Build history of the part. All positions in model axes, mm. Give positions to 0.01 mm unless a question says otherwise; leave off trailing zeros. Order: outer loops, then holes, each group sorted by start corner. A loop starts at its lowest first (then second) coordinate and runs counter-clockwise, first axis right, second up. Notation, with made-up numbers: (-23, 2) - (9, 2) arc R14 ccw to (9, 8) - close; hole circle Ø11 at (26.5, 38.5). An arc over 180 degrees is marked (long way). Use a Markdown table: item, result.
from build123d import *

# Parameters (mm, degrees)
BOSS_EXTRUDE1_DEPTH     = 6
SKETCH2_OUTSIDE_W       = 77.868
SKETCH2_OUTSIDE_H       = 81.89
SKETCH2_OUTSIDE_R       = 13
CUT_EXTRUDE1_DEPTH      = 12
CUT_EXTRUDE1_DRAFT      = -60
MIRROR1_COPY_1_SKETCH_W = 77.868
MIRROR1_COPY_1_SKETCH_H = 81.89
MIRROR1_COPY_1_SKETCH_R = 13
MIRROR1_COPY_1_DEPTH    = 12
MIRROR1_COPY_1_DRAFT    = -60
SKETCH3_R               = 10
CUT_EXTRUDE2_DEPTH      = 24.202011407
CHAMFER1_SIZE           = 1


with BuildPart() as part:
    # Sketch1 → Boss-Extrude1 (new, symmetric)
    with BuildSketch(Plane(origin=(0, 0, 0), x_dir=(1, 0, 0), z_dir=(0, 1, 0))):
        Polygon((13, 7.505553499), (0, 15.011106999), (-13, 7.505553499), (-13, -7.505553499), (0, -15.011106999), (13, -7.505553499), align=None)
    extrude(amount=BOSS_EXTRUDE1_DEPTH, both=True)


with BuildPart() as cut_extrude1_tool:
    # Sketch2 outside → Cut-Extrude1 (with draft: the straight prism first)
    with BuildSketch(Plane(origin=(0, 6, 0), x_dir=(1, 0, 0), z_dir=(0, 1, 0))):
        Rectangle(SKETCH2_OUTSIDE_W, SKETCH2_OUTSIDE_H)
        Circle(SKETCH2_OUTSIDE_R, mode=Mode.SUBTRACT)
    extrude(amount=-CUT_EXTRUDE1_DEPTH)
    # Cut-Extrude1: the draft: its side faces are tilted about the plane it starts from
    cut_extrude1_sides = [cut_extrude1_tool.faces().sort_by_distance(p)[0] for p in [
        (0, 0, 40.945),
        (38.934, 0, 0),
        (0, 0, -40.945),
        (-38.934, 0, 0),
        (-13, 0, 0),
    ]]
    draft(cut_extrude1_sides, Plane(origin=(0, 6, 0), x_dir=(1, 0, 0), z_dir=(0, 1, 0)), CUT_EXTRUDE1_DRAFT)


with BuildPart() as part_1:
    add(part.part)

    # Cut-Extrude1: cut by cut_extrude1_tool
    add(cut_extrude1_tool.part, mode=Mode.SUBTRACT)


with BuildPart() as mirror1_copy_1_tool:
    # Mirror1 copy 1 sketch → Mirror1 copy 1 (with draft: the straight prism first)
    with BuildSketch(Plane.XZ.offset(6)):
        Rectangle(MIRROR1_COPY_1_SKETCH_W, MIRROR1_COPY_1_SKETCH_H)
        Circle(MIRROR1_COPY_1_SKETCH_R, mode=Mode.SUBTRACT)
    extrude(amount=-MIRROR1_COPY_1_DEPTH)
    # Mirror1 copy 1: the draft: its side faces are tilted about the plane it starts from
    mirror1_copy_1_sides = [mirror1_copy_1_tool.faces().sort_by_distance(p)[0] for p in [
        (0, 0, 40.945),
        (38.934, 0, 0),
        (0, 0, -40.945),
        (-38.934, 0, 0),
        (-13, 0, 0),
    ]]
    draft(mirror1_copy_1_sides, Plane.XZ.offset(6), MIRROR1_COPY_1_DRAFT)


with BuildPart() as part_2:
    add(part_1.part)

    # Mirror1 copy 1: cut by mirror1_copy_1_tool
    add(mirror1_copy_1_tool.part, mode=Mode.SUBTRACT)

    # Sketch3 → Cut-Extrude2 (cut, through all)
    with BuildSketch(Plane(origin=(0, 6, 0), x_dir=(1, 0, 0), z_dir=(0, 1, 0))):
        with Locations(Location((0, 0, 0), (0, 0, 270))):
            Circle(SKETCH3_R)
    extrude(amount=-CUT_EXTRUDE2_DEPTH, mode=Mode.SUBTRACT)

    # Chamfer1
    chamfer1_edges = [part_2.edges().sort_by_distance(p)[0] for p in [
        (0, -6, -10),
        (0, 6, -10),
    ]]
    chamfer(chamfer1_edges, length=CHAMFER1_SIZE)


solid = part_2.part
1) Slice it at A-A (y = 2.25). Write the cut outline in (x, z), and give its area (3 significant figures).
Computed:
| item | result |
|---|---|
| outline | (-13, -7.51) - (0, -15.01) - (13, -7.51) - (13, 7.51) - (0, 15.01) - (-13, 7.51) - close; hole circle Ø20 at (0, 0) |
| area | 271 mm² |
2) Wall check: line 1 (X direction, y = -0.5, z = 0); line 2 (X direction, y = -3, z = 6.5); line 3 (Z direction, x = 8.5, y = 1). Give the ranges that are in metal, low to high. Write a range as from..to.
Computed:
| item | result |
|---|---|
| line 1 | x = -13..-10, 10..13 |
| line 2 | x = -13..-7.6, 7.6..13 |
| line 3 | z = -10.1..-5.27, 5.27..10.1 |
3) Two-plate mould, pull along Z, no slides. Class faces 1 (the cylindrical face through (-9.76, 0.07, -2.17)), 2 (the flat face through (-11, -6, -3)), 3 (the conical face through (-11.66, 5.72, -6.77)): +Z half, -Z half, draft (parallel to the pull), parting line (faces both ways), or undercut.
Computed:
| item | result |
|---|---|
| face 1 | undercut |
| face 2 | draft |
| face 3 | -Z half |
4) Pin check, flat tips, straight feed: P1, Ø6, axis at x = -6, y = -3, coming from the +Z side; P2, Ø5, axis at x = 4, y = 4.5, coming from the -Z side; P3, Ø3, axis at x = 4, y = 0.5, coming from the -Z side. Stop position of each tip, or through.
Computed:
| item | result |
|---|---|
| P1 | stops at z = 13.28 |
| P2 | stops at z = -14.15 |
| P3 | stops at z = -13.57 |
